Here's how the part is built. I have some questions about the finished solid (model axes, mm). A direction names the side the tool comes from. Round coordinates to 2 decimals unless told otherwise and drop trailing zeros. Order: outer loops, then holes, each group sorted by start corner. A loop starts at its lowest first (then second) coordinate and runs counter-clockwise, first axis right, second up. Notation, with made-up numbers: M 65.25,13 L 85.25,13 A10 ccw 85.25,29 Z; hole C 23.5,77.25 d4. An arc over 180 degrees is marked long. Write each question's results on one line, items separated by ' | '. Start each with the question number.
```python
from build123d import *

# Parameters (mm, degrees)
SKETCH_2_R             = 3
CUT_EXTRUDE_1_DEPTH    = 6
CHAMFER_1_SIZE         = 1
CHAMFER_1_SIZE2        = 1.732050808
SKETCH_3_W             = 11
SKETCH_3_H             = 1.5
CUT_EXTRUDE_3_DEPTH    = 6
CHAMFER_2_SIZE         = 0.2
HOLE_WIZARD_M2_1_D     = 2.4
HOLE_WIZARD_M2_1_DEPTH = 10
HOLE_WIZARD_M2_1_TIP   = 0.721032743


with BuildPart() as part:
    # 草图1 → 旋转1 (revolve)
    with BuildSketch(Plane.XY, mode=Mode.PRIVATE) as revolve_1_sk:
        Polygon((0, 0), (-2, 0), (-2, -25), (-4, -25), (-4, -28.5), (-4.5, -28.5), (-4.5, -32.5), (0, -32.5), align=None)
    revolve(revolve_1_sk.sketch.rotate(Axis((0, 0, 0), (0, -1, 0)), 270), axis=Axis((0, 0, 0), (0, -1, 0)))

    # 草图2 → 切除-拉伸1 (cut)
    with BuildSketch(Plane.XZ.offset(32.5)):
        with Locations(Location((0, 0, 0), (0, 0, 270))):
            Circle(SKETCH_2_R)
    extrude(amount=-CUT_EXTRUDE_1_DEPTH, mode=Mode.SUBTRACT)

    # 倒角1
    chamfer_1_edges = [part.edges().sort_by_distance(p)[0] for p in [
        (0, -32.5, 3),
    ]]
    chamfer_1_side = [part.faces().sort_by_distance(p)[0] for p in [
        (0, -32.5, -4.372720779),
    ]]
    chamfer(chamfer_1_edges, length=CHAMFER_1_SIZE, length2=CHAMFER_1_SIZE2, reference=chamfer_1_side[0])

    # 草图3 → 切除-拉伸3 (cut)
    with BuildSketch(Plane.XZ.offset(32.5)):
        Rectangle(SKETCH_3_W, SKETCH_3_H)
    extrude(amount=-CUT_EXTRUDE_3_DEPTH, mode=Mode.SUBTRACT)

    # 倒角2
    chamfer_2_edges = [part.edges().sort_by_distance(p)[0] for p in [
        (0, 0, -2),
    ]]
    chamfer(chamfer_2_edges, length=CHAMFER_2_SIZE)

    # M2 间隙孔1
    with Locations(Plane(origin=(-1.999095, -18, -0.060159626), x_dir=(0.030079813167, 0, -0.999547500042), z_dir=(-0.999547500042, 0, -0.030079813167))):
        with Locations((0, 0)):
            Hole(HOLE_WIZARD_M2_1_D / 2, depth=HOLE_WIZARD_M2_1_DEPTH)
            with Locations((0, 0, -(HOLE_WIZARD_M2_1_DEPTH + HOLE_WIZARD_M2_1_TIP / 2))):  # 118° drill point
                Cone(0, HOLE_WIZARD_M2_1_D / 2, HOLE_WIZARD_M2_1_TIP, mode=Mode.SUBTRACT)


solid = part.part
```
(1) On a 3-axis mill with a long thin cutter (end or side, diameter ignored), from which of +Z, -Z, +X, -X, +Y, -Y can I reach the whole of each face in a straight line? I mean faces 4 (the flat face through (0.31, -28.5, -4.14)), 5 (the cylindrical face through (-0.1, -30.5, -4.5)), 6 (the cylindrical face through (3.549, -26.774, 1.846)), 7 (the conical face through (-0.06, -31.24, -3.27)), 8 (the flat face through (4, -30, -0.75)). Say none if no direction works.
(2) I want a section at A-A on y = -21.5. Write out the boundary of the cut face in (x, z), and give its area (3 significant figures).
(3) If we mould it in two halves opening along Y, with no side actions, what happens to faces 1 (the flat face through (0.3, -28.5, 4.2)), 2 (the cylindrical face through (0.064, -18.053, -1.197)), 3 (the flat face through (-4, -30, -0.75))? For each: pulls with the +Y half, pulls with the -Y half, needs draft (parallel to the pull), parting line crosses it, or undercut.
(4) Please list where these lines run through material, in increasing order: line 1 (Y direction, x = -1.25, z = 0); line 2 (Z direction, x = -3.25, y = -27); line 3 (Z direction, x = -1.5, y = -17).
(5) I'm going to push flat-ended pins straight in: pin 1 Ø3 at (y, z) = (-9.5, -0.5) entering from -X; pin 2 Ø0.8 at (x, y) = (3.5, -29.5) entering from +Z; pin 3 Ø3 at (x, z) = (-0.5, -3.5) entering from +Y; pin 4 Ø4 at (x, z) = (-1, 2) entering from +Y. Where does each tip first touch, or does it pass through?
Solutions:
1) face 4: -Z, +Y | face 5: -Z, +Y, -Y | face 6: +Y | face 7: -Y | face 8: +X, -X, -Y
2) outline: C 0,0 d4 | area: 12.6 mm^2
3) face 1: pulls with the +Y half | face 2: undercut | face 3: needs draft
4) line 1: -26.5 to -19.2, -16.8 to 0 | line 2: -2.33 to -0.75, 0.75 to 2.33 | line 3: -1.32 to -0.71, 0.62 to 1.32
5) pin 1: x = -2 | pin 2: z = 3.26 | pin 3: y = -25 | pin 4: y = 0
